from build123d import *

# Parameters (mm, degrees)
SKETCH1_W               = 5
SKETCH1_H               = 5
SKETCH1_W_2             = 4.5
SKETCH1_H_2             = 4.5
BOSS_EXTRUDE1_DEPTH     = 25.5
CUT_EXTRUDE1_DEPTH      = 27.105554964
CUT_EXTRUDE1_DEPTH_BACK = 27.105554964
SKETCH2_W               = 0.5
SKETCH2_H               = 10


with BuildPart() as part:
    # Sketch1 → Boss-Extrude1 (new body)
    with BuildSketch(Plane(origin=(0, 0, 0), x_dir=(1, 0, 0), z_dir=(0, 1, 0))):
        Rectangle(SKETCH1_W, SKETCH1_H)
        Rectangle(SKETCH1_W_2, SKETCH1_H_2, mode=Mode.SUBTRACT)
    extrude(amount=BOSS_EXTRUDE1_DEPTH)

    # Sketch2 → Cut-Extrude1 (cut, two sides: drawn at the far end of the back side and taken through both)
    with BuildSketch(Plane.XY.offset(2.5).offset(-CUT_EXTRUDE1_DEPTH_BACK)):
        with Locations((1.75, 7.5)):
            Rectangle(SKETCH2_W, SKETCH2_H)
    extrude(amount=CUT_EXTRUDE1_DEPTH + CUT_EXTRUDE1_DEPTH_BACK, mode=Mode.SUBTRACT)


solid = part.part
Verification items for the finished model (mm, model axes). A direction names the side the tool comes from. Coordinates: 2 decimals unless noted, no trailing zeros. Write each loop counter-clockwise with the first axis right and the second up, starting at its lowest first coordinate (ties: lowest second). Pieces come first, ordered by that corner, then holes. Notation, with made-up numbers: M 5,76 L 12,76 A14 cw 12,89 Z; hole C -6.75,79.5 d1. An arc over 180 degrees is marked long. Use CSV: the item, a comma, the result in double quotes.
Q1. Section check C-C, the plane y = 2.25. Enter the section's corners in (x, z).
Computed values:
outline,"M -2.5,-2.5 L 2.5,-2.5 L 2.5,2.5 L -2.5,2.5 Z; hole M -2.25,-2.25 L 2.25,-2.25 L 2.25,2.25 L -2.25,2.25 Z"
Q2. Section check D-D, the plane y = 10.75. Enter the section's corners in (x, z), and give its area (3 significant figures).
Computed values:
outline,"M -2.5,-2.5 L 1.5,-2.5 L 1.5,-2.25 L -2.25,-2.25 L -2.25,2.25 L 1.5,2.25 L 1.5,2.5 L -2.5,2.5 Z; M 2,-2.5 L 2.5,-2.5 L 2.5,2.5 L 2,2.5 L 2,2.25 L 2.25,2.25 L 2.25,-2.25 L 2,-2.25 Z"
area,"4.50 mm²"
Q3. Section check A-A, the plane z = -0.05. Enter the section's corners in (x, y), and give its area (4 significant figures).
Computed values:
outline,"M -2.5,0 L -2.25,0 L -2.25,25.5 L -2.5,25.5 Z; M 2.25,0 L 2.5,0 L 2.5,25.5 L 2.25,25.5 Z"
area,"12.75 mm²"
Q4. Thickness scan on line 1 along X through (y, z) = (11, -0.8). Record the ranges inside material, lowest first. Write a range as [from, to].
Computed values:
line 1,"[-2.5, -2.25], [2.25, 2.5]"
Q5. Set-up check for faces 5 (the flat face through (0, 13, -2.5)), 6 (the flat face through (0, 13, -2.25)): record each of +Z, -Z, +X, -X, +Y, -Y from which the full face is reachable in a straight line by a thin tool's end or side.
Computed values:
face 5,"-Z, +X, -X, +Y, -Y"
face 6,"+Y, -Y"
Q6. Section check B-B, the plane x = -0.45. Enter the section's corners in (y, z), and give its area (4 significant figures).
Computed values:
outline,"M 0,-2.5 L 25.5,-2.5 L 25.5,-2.25 L 0,-2.25 Z; M 0,2.25 L 25.5,2.25 L 25.5,2.5 L 0,2.5 Z"
area,"12.75 mm²"
Q7. Mould release check, pull along X, two halves, no side actions. Record for faces 1 (the flat face through (-2.5, 13, 0)), 2 (the flat face through (0, 13, 2.25)), 3 (the flat face through (2.5, 13, 0)), 4 (the flat face through (0, 13, 2.5)): pulls with the +X half, pulls with the -X half, needs draft (parallel to the pull), parting line crosses it, or undercut.
Computed values:
face 1,"pulls with the -X half"
face 2,"undercut"
face 3,"pulls with the +X half"
face 4,"needs draft"
